CAD build for the part. Positions are in the model's coordinates, mm. A direction names the side the tool comes from. Round coordinates to 2 decimals unless told otherwise and drop trailing zeros. Answer as a JSON object with one key per item and string values. Group by question number.
```python
from build123d import *

# Parameters (mm, degrees)
SKIZZE1_W                       = 80
SKIZZE1_H                       = 195
AUFSATZ_LINEAR_AUSTRAGEN1_DEPTH = 10
SKIZZE2_R                       = 3.015
SKIZZE2_R_2                     = 15.25
SCHNITT_LINEAR_AUSTRAGEN1_DEPTH = 10
SKIZZE3_R                       = 2.5
SCHNITT_LINEAR_AUSTRAGEN2_DEPTH = 5
SKIZZE6_R                       = 1.25
SCHNITT_LINEAR_AUSTRAGEN4_DEPTH = 5
SKIZZE7_R                       = 1
SCHNITT_LINEAR_AUSTRAGEN5_DEPTH = 20
SCHNITT_LINEAR_START            = -30
SKIZZE8_R                       = 1
SCHNITT_LINEAR_AUSTRAGEN6_DEPTH = 30


with BuildPart() as part:
    # Skizze1 → Aufsatz-Linear austragen1 (new body)
    with BuildSketch(Plane.XY):
        with Locations((-29.059385344, -27.400468384)):
            Rectangle(SKIZZE1_W, SKIZZE1_H)
    extrude(amount=-AUFSATZ_LINEAR_AUSTRAGEN1_DEPTH)

    # Skizze2 → Schnitt-Linear austragen1 (cut)
    with BuildSketch(Plane(origin=(0, 0, -10), x_dir=(-1, 0, 0), z_dir=(0, 0, -1))):
        with Locations((18.659385344, -12.400468384)):
            Circle(SKIZZE2_R)
        with Locations((48.659385344, -12.400468384)):
            Circle(SKIZZE2_R)
        with Locations((18.659385344, -42.400468384)):
            Circle(SKIZZE2_R)
        with Locations((48.659385344, -42.400468384)):
            Circle(SKIZZE2_R)
        with Locations((33.659385344, -27.400468384)):
            Circle(SKIZZE2_R_2)
    extrude(amount=-SCHNITT_LINEAR_AUSTRAGEN1_DEPTH, mode=Mode.SUBTRACT)

    # Skizze3 → Schnitt-Linear austragen2 (cut)
    with BuildSketch(Plane(origin=(0, 0, -10), x_dir=(-1, 0, 0), z_dir=(0, 0, -1))):
        with Locations((29.059385344, 65.099531616)):
            Circle(SKIZZE3_R)
        with Locations((-5.940614656, 65.099531616)):
            Circle(SKIZZE3_R)
        with Locations((64.059385344, 65.099531616)):
            Circle(SKIZZE3_R)
        with Locations((29.059385344, -119.900468384)):
            Circle(SKIZZE3_R)
        with Locations((-5.940614656, -119.900468384)):
            Circle(SKIZZE3_R)
        with Locations((64.059385344, -119.900468384)):
            Circle(SKIZZE3_R)
        with Locations((-5.940614656, 42.599531616)):
            Circle(SKIZZE3_R)
        with Locations((-5.940614656, -27.400468384)):
            Circle(SKIZZE3_R)
        with Locations((-5.940614656, -97.400468384)):
            Circle(SKIZZE3_R)
        with Locations((64.059385344, -97.400468384)):
            Circle(SKIZZE3_R)
        with Locations((64.059385344, -27.400468384)):
            Circle(SKIZZE3_R)
        with Locations((64.059385344, 42.599531616)):
            Circle(SKIZZE3_R)
    extrude(amount=-SCHNITT_LINEAR_AUSTRAGEN2_DEPTH, mode=Mode.SUBTRACT)

    # Skizze6 → Schnitt-Linear austragen4 (cut)
    with BuildSketch(Plane.XY):
        with Locations((-64.059385344, 65.099531616)):
            Circle(SKIZZE6_R)
        with Locations((-29.059385344, 65.099531616)):
            Circle(SKIZZE6_R)
        with Locations((5.940614656, 65.099531616)):
            Circle(SKIZZE6_R)
        with Locations((-64.059385344, 42.599531616)):
            Circle(SKIZZE6_R)
        with Locations((-64.059385344, -27.400468384)):
            Circle(SKIZZE6_R)
        with Locations((-64.059385344, -97.400468384)):
            Circle(SKIZZE6_R)
        with Locations((-64.059385344, -119.900468384)):
            Circle(SKIZZE6_R)
        with Locations((5.940614656, -119.900468384)):
            Circle(SKIZZE6_R)
        with Locations((5.940614656, -97.400468384)):
            Circle(SKIZZE6_R)
        with Locations((5.940614656, -27.400468384)):
            Circle(SKIZZE6_R)
        with Locations((5.940614656, 42.599531616)):
            Circle(SKIZZE6_R)
    extrude(amount=-SCHNITT_LINEAR_AUSTRAGEN4_DEPTH, mode=Mode.SUBTRACT)

    # Skizze7 → Schnitt-Linear austragen5 (cut)
    with BuildSketch(Plane.ZY.offset(69.059385344)):
        with Locations((-5, -12.400468384)):
            Circle(SKIZZE7_R)
        with Locations((-5, -42.400468384)):
            Circle(SKIZZE7_R)
    extrude(amount=-SCHNITT_LINEAR_AUSTRAGEN5_DEPTH, mode=Mode.SUBTRACT)

    # Skizze8 → Schnitt-Linear austragen6 (cut)
    with BuildSketch(Plane(origin=(10.940614656, 0, 0), x_dir=(0, 0, -1), z_dir=(1, 0, 0)).offset(SCHNITT_LINEAR_START)):
        with Locations(Location((5, -12.400468384, 0), (0, 0, 180))):
            Circle(SKIZZE8_R)
        with Locations(Location((5, -42.400468384, 0), (0, 0, 180))):
            Circle(SKIZZE8_R)
    extrude(amount=SCHNITT_LINEAR_AUSTRAGEN6_DEPTH, mode=Mode.SUBTRACT)


solid = part.part
```
Item 1: Two-plate mould, pull along Y, no slides. Class faces 1 (the face through (-30, -124.9, -5)), 2 (the face through (-69.059, -29, -5)), 3 (the face through (-65, -26, -5)): +Y half, -Y half, draft (parallel to the pull), parting line (faces both ways), or undercut.
Item 2: 3-axis set-ups, long thin cutter, end or side, ignore diameter. For faces 4 (the face through (-21.535, -41.495, -5.07)), 5 (the face through (6.48, -29.84, -7.54)): which of +Z, -Z, +X, -X, +Y, -Y reach the whole face in a straight line?
Item 3: Flat gauge pins, fed straight in: pin 1 Ø5.5 at (x, y) = (-48.66, -12.4) entering from +Z; pin 2 Ø1.2 at (y, z) = (-42.4, -5) entering from +X; pin 3 Ø2.5 at (x, y) = (-65, 65) entering from -Z. Where does each tip first touch, or does it go through?
Item 4: Drill centre lines: line 1 (X direction, y = -98, z = -4.5); line 2 (X direction, y = -28.5, z = -4.5); line 3 (Y direction, x = -50, z = -6.5). Where is each one in solid material? Low to high. Write a range as [from, to].
Response values:
{
 "1": {"face 1": "-Y half", "face 2": "draft", "face 3": "undercut"},
 "2": {"face 4": "+Z, -Z", "face 5": "-Z"},
 "3": {"pin 1": "through", "pin 2": "x = -21.61", "pin 3": "z = -5"},
 "4": {"line 1": "[-69.06, -65.16], [-62.96, 4.84], [7.04, 10.94]", "line 2": "[-69.06, -64.65], [-63.46, -48.87], [-18.45, 5.35], [6.54, 10.94]", "line 3": "[-124.9, -45.1], [-39.7, -15.1], [-9.7, 70.1]"}
}
